```python
from build123d import *

# Parameters (mm, degrees)
SKETCH1_R                 = 6.35
BOSS_EXTRUDE1_DEPTH       = 12.7
M3X0_5_TAPPED_HOLE1_D     = 2.5
F_6_32_TAPPED_HOLE1_D     = 2.7051
F_6_32_TAPPED_HOLE1_DEPTH = 9.398
F_6_32_TAPPED_HOLE1_TIP   = 0.81269403
CHAMFER1_SIZE             = 6.35
CHAMFER1_SIZE2            = 3.81


with BuildPart() as part:
    # Sketch1 → Boss-Extrude1 (new body)
    with BuildSketch(Plane.XY):
        Circle(SKETCH1_R)
    extrude(amount=BOSS_EXTRUDE1_DEPTH)

    # M3x0.5 Tapped Hole1 (through all)
    with Locations(Plane.XY.offset(12.7)):
        with Locations((0, 0)):
            Hole(M3X0_5_TAPPED_HOLE1_D / 2)

    # #6-32 Tapped Hole1
    with Locations(Plane(origin=(0, 0, 0), x_dir=(-1, 0, 0), z_dir=(0, 0, -1))):
        with Locations((0, 0)):
            Hole(F_6_32_TAPPED_HOLE1_D / 2, depth=F_6_32_TAPPED_HOLE1_DEPTH)
            with Locations((0, 0, -(F_6_32_TAPPED_HOLE1_DEPTH + F_6_32_TAPPED_HOLE1_TIP / 2))):  # 118° drill point
                Cone(0, F_6_32_TAPPED_HOLE1_D / 2, F_6_32_TAPPED_HOLE1_TIP, mode=Mode.SUBTRACT)

    # Chamfer1
    chamfer1_edges = [part.edges().sort_by_distance(p)[0] for p in [
        (-6.35, 0, 12.7),
    ]]
    chamfer1_side = [part.faces().sort_by_distance(p)[0] for p in [
        (-6.35, 0, 6.35),
    ]]
    chamfer(chamfer1_edges, length=CHAMFER1_SIZE, length2=CHAMFER1_SIZE2, reference=chamfer1_side[0])


solid = part.part
```
CAD build for the part. Positions are in the model's coordinates, mm. Coordinates: 2 decimals unless noted, no trailing zeros. Write each loop counter-clockwise with the first axis right and the second up, starting at its lowest first coordinate (ties: lowest second). Pieces come first, ordered by that corner, then holes. Notation, with made-up numbers: (40, 83.5) -> (68, 83.5) arc R23 ccw to (68, 116.5) -> close; hole circle Ø6 at (3.5, 67). An arc over 180 degrees is marked (long way). Use CSV: the item, a comma, the result in double quotes. Start each with the question number.
Item 1: Drop flat-ended pins along their axis: P1, Ø1.5, axis at x = 2.5, z = 3, coming from the +Y side; P2, Ø4, axis at x = -3, z = 7.5, coming from the +Y side. Give the stop position or say it passes through.
Item 2: Band-saw the part on C-C, the plane z = 1.5. Write the cut outline in (x, y).
Item 3: Wall check: probe 1 along X at (y, z) = (0, 6.5); probe 2 along Y at (x, z) = (0, 11.4); probe 3 along X at (y, z) = (0, 10.35). Give the ranges that are in metal, low to high.
Item 4: Band-saw the part on A-A, the plane y = 0. Write the cut outline in (x, z).
Item 5: Two-plate mould, pull along X, no slides. Class faces 1 (the cylindrical face through (1.29, 0.41, 4.76)), 2 (the flat face through (-1, -1, 12.7)), 3 (the cylindrical face through (-1.38, -6.2, 3.13)), 4 (the cylindrical face through (0.27, -1.22, 11.06)): +X half, -X half, draft (parallel to the pull), parting line (faces both ways), or undercut.
Response values:
1,P1,"stops at y = 6.1"
1,P2,"stops at y = 6.2"
2,outline,"circle Ø12.7 at (0, 0); hole circle Ø2.71 at (0, 0)"
3,probe 1,"x = -6.26 to -1.35, 1.35 to 6.26"
3,probe 2,"y = -3.32 to -1.25, 1.25 to 3.32"
3,probe 3,"x = -3.95 to -1.25, 1.25 to 3.95"
4,outline,"(-6.35, 0) -> (-1.35, 0) -> (-1.35, 9.4) -> (-1.25, 9.46) -> (-1.25, 12.7) -> (-2.54, 12.7) -> (-6.35, 6.35) -> close; (1.25, 9.46) -> (1.35, 9.4) -> (1.35, 0) -> (6.35, 0) -> (6.35, 6.35) -> (2.54, 12.7) -> (1.25, 12.7) -> close"
5,face 1,"undercut"
5,face 2,"draft"
5,face 3,"parting line"
5,face 4,"undercut"
